Source: CAD feature listing. Evaluate the final solid. Frame: model axes, mm. A direction names the side the tool comes from. Give positions to 0.01 mm unless a question says otherwise; leave off trailing zeros. Loops run counter-clockwise (first coordinate to the right, second up) from the corner with the lowest first, then second, coordinate; pieces in that order, holes last. Notation, with made-up numbers: (80, 24) -> (121, 24) arc R18 cw to (121, 42) -> close; hole circle Ø6 at (-20, 21.25). An arc over 180 degrees is marked (long way). Return JSON: item names as keys, results as strings. Group by question number.
```python
from build123d import *

# Parameters (mm, degrees)
F0_R            = 35
F0_R_2          = 14
F1_DEPTH        = 8
F2_DEPTH        = 4
F4_D            = 4.4
F4_CBORE_D      = 8.25
F4_CBORE_DEPTH  = 4
F4_COPIES_COUNT = 4
F5_D            = 5.5
F5_CBORE_D      = 9.75
F5_CBORE_DEPTH  = 5
F5_COPIES_COUNT = 4


# Not quite as in the source:
# - a pattern or mirror of a feature is missing from the dataset's text; its kind, count and spacing are read off the source's solid


with BuildPart() as f1:
    # F0 (on Front) → F1 (new body)
    with BuildSketch(Plane.XZ):
        Circle(F0_R)
        Circle(F0_R_2, mode=Mode.SUBTRACT)
        Circle(F0_R_2)
    extrude(amount=F1_DEPTH)

    # F0 (on Front) → F2 (join)
    with BuildSketch(Plane.XZ):
        Circle(F0_R_2)
    extrude(amount=-F2_DEPTH)

    # F4 (through all)
    with Locations(Plane.XZ.offset(8)):
        with Locations((12.0208152802, 12.0208152802)):
            f4 = CounterBoreHole(F4_D / 2, F4_CBORE_D / 2, F4_CBORE_DEPTH)

    # F4_copies: F4 ×4 about axis
    f4_copies_axis = Axis((0, 0, 0), (0, 1, 0))
    for i in range(1, F4_COPIES_COUNT):
        add(f4.rotate(f4_copies_axis, i * 360 / F4_COPIES_COUNT), mode=Mode.SUBTRACT)

    # F5 (through all)
    with Locations(Plane(origin=(0, 0, 0), x_dir=(1, 0, 0), z_dir=(0, 1, 0))):
        with Locations((0, -28)):
            f5 = CounterBoreHole(F5_D / 2, F5_CBORE_D / 2, F5_CBORE_DEPTH)

    # F5_copies: F5 ×4 about axis
    f5_copies_axis = Axis((0, 0, 0), (0, 1, 0))
    for i in range(1, F5_COPIES_COUNT):
        add(f5.rotate(f5_copies_axis, i * 360 / F5_COPIES_COUNT), mode=Mode.SUBTRACT)


solid = f1.part
```
1) Mould query, pull axis X, two halves, no side actions, for faces 4 (the face through (-25.273, -6.521, 0.358)), 5 (the face through (-28, -4, -21)), 6 (the face through (0, -8, 0)). Classes: released by +X, released by -X, zero draft, split by the parting line, or undercut.
2) Cut plane A-A on z = 0. Return loops of the section in (x, y) (3 decimals), then the cut area to 4 significant figures.
3) Reachability of faces 1 (the face through (15.5, -6.03, -14.24)), 2 (the face through (-32.76, -2.46, -1.06)), 3 (the face through (-12.498, -1.972, -9.873)) from +Z, -Z, +X, -X, +Y, -Y: full face, straight path, thin tool, end or side. Return the list, or none.
4) Cut plane C-C on z = 28. Return loops of the section in (x, y) (3 decimals).
5) Cut plane B-B on x = -28. Return loops of the section in (y, z) (3 decimals).
6) Cut plane D-D on y = -7. Count the separate pieces of the cut face and the enclosed holes in it, then the cut area to 3 significant figures.
7) Contact query for flat-ended pins moving along their axis: P1, Ø3.5, axis at x = 0, z = 28, coming from the +Y side; P2, Ø2, axis at x = 16, y = -3, coming from the -Z side; P3, Ø4, axis at x = 21.5, y = 1.5, coming from the -Z side; P4, Ø6, axis at x = 23.5, y = -2.5, coming from the +Z side. Output: stop coordinate, or through.
8) Material intervals for line 1 (Z direction, x = -10.5, y = -4.75); line 2 (X direction, y = -3.75, z = -3); line 3 (Z direction, x = 13.5, y = -6.75), sorted ascending.
Calculated:
{
 "1": {"face 4": "undercut", "face 5": "split by the parting line", "face 6": "zero draft"},
 "2": {"outline": "(-35, -8) -> (-30.75, -8) -> (-30.75, -5) -> (-32.875, -5) -> (-32.875, 0) -> (-35, 0) -> close; (-25.25, -8) -> (25.25, -8) -> (25.25, -5) -> (23.125, -5) -> (23.125, 0) -> (14, 0) -> (14, 4) -> (-14, 4) -> (-14, 0) -> (-23.125, 0) -> (-23.125, -5) -> (-25.25, -5) -> close; (30.75, -8) -> (35, -8) -> (35, 0) -> (32.875, 0) -> (32.875, -5) -> (30.75, -5) -> close", "area": "541.5 mm2"},
 "3": {"face 1": "-Y", "face 2": "+Y", "face 3": "+Y, -Y"},
 "4": {"outline": "(-21, -8) -> (-2.75, -8) -> (-2.75, -5) -> (-4.875, -5) -> (-4.875, 0) -> (-21, 0) -> close; (2.75, -8) -> (21, -8) -> (21, 0) -> (4.875, 0) -> (4.875, -5) -> (2.75, -5) -> close"},
 "5": {"outline": "(-8, -21) -> (0, -21) -> (0, -4.875) -> (-5, -4.875) -> (-5, -2.75) -> (-8, -2.75) -> close; (-8, 2.75) -> (-5, 2.75) -> (-5, 4.875) -> (0, 4.875) -> (0, 21) -> (-8, 21) -> close"},
 "6": {"separate pieces": "1", "enclosed holes": "8", "area": "3,540 mm2"},
 "7": {"P1": "through", "P2": "z = -31.62", "P3": "z = -28.6", "P4": "z = 28.37"},
 "8": {"line 1": "-33.39 to -15.86, -8.19 to 8.19, 15.86 to 33.39", "line 2": "-34.87 to -31.84, -24.16 to 24.16, 31.84 to 34.87", "line 3": "-32.29 to -15.87, -8.17 to 8.17, 15.87 to 32.29"}
}
